Read the model definition and answer for the solid it produces. Units are mm, in the model's axes. Face numbers are marked on the shaded views. A direction names the side the tool comes from. Give positions to 0.01 mm unless a question says otherwise; leave off trailing zeros. Order: outer loops, then holes, each group sorted by start corner. A loop starts at its lowest first (then second) coordinate and runs counter-clockwise, first axis right, second up.
```python
from build123d import *

# Parameters (mm, degrees)
S_BOX1_W       = 20
S_BOX1_H       = 2.5
BOSS_1_DEPTH   = 42
S_BOX2_W       = 30.4
S_BOX2_H       = 24
BOSS_2_DEPTH   = 27.6
S_CUT3_W       = 30.6
S_CUT3_H       = 13
POCKET_3_DEPTH = 23.6
S_CUT4_W       = 23
S_CUT4_H       = 4
POCKET_4_DEPTH = 23.7
S_HOLE5_R      = 1.5
HOLE_5_DEPTH   = 2.7


with BuildPart() as part:
    # S_box1 → Boss_1 (new body)
    with BuildSketch(Plane.XY.offset(-34)):
        with Locations((0, 2.75)):
            Rectangle(S_BOX1_W, S_BOX1_H)
    extrude(amount=BOSS_1_DEPTH)

    # S_box2 → Boss_2 (add)
    with BuildSketch(Plane.XY.offset(-35.4)):
        with Locations((-3.8, 13.5)):
            Rectangle(S_BOX2_W, S_BOX2_H)
    extrude(amount=BOSS_2_DEPTH)

    # S_cut3 → Pocket_3 (cut)
    with BuildSketch(Plane.XY.offset(-33.4)):
        with Locations((-3.8, 17)):
            Rectangle(S_CUT3_W, S_CUT3_H)
    extrude(amount=POCKET_3_DEPTH, mode=Mode.SUBTRACT)

    # S_cut4 → Pocket_4 (cut)
    with BuildSketch(Plane.XY.offset(-35.5)):
        with Locations((-3.5, 6.5)):
            Rectangle(S_CUT4_W, S_CUT4_H)
    extrude(amount=POCKET_4_DEPTH, mode=Mode.SUBTRACT)

    # S_hole5 → Hole_5 (cut)
    with BuildSketch(Plane(origin=(0, 1.4, 0), x_dir=(1, 0, 0), z_dir=(0, 1, 0))):
        with Locations(Location((0, 0, 0), (0, 0, 90))):
            Circle(S_HOLE5_R)
    extrude(amount=HOLE_5_DEPTH, mode=Mode.SUBTRACT)


solid = part.part
```
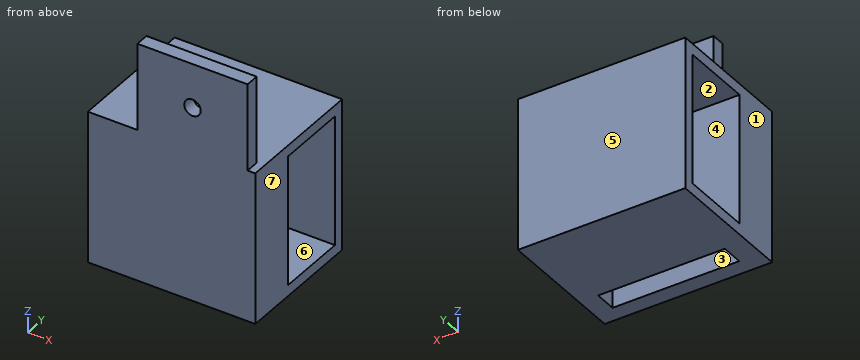
1) The part is cut by section A-A on y = 17. Determine the outline of the cut face in (x, z), and give its area (3 significant figures).
Final values:
outline: (-19, -35.4) - (11.4, -35.4) - (11.4, -33.4) - (-19, -33.4) - close; (-19, -9.8) - (11.4, -9.8) - (11.4, -7.8) - (-19, -7.8) - close
area: 122 mm2
2) The part is cut by section B-B on x = 0. Determine the outline of the cut face in (y, z), and give its area (3 significant figures).
Final values:
outline: (1.5, -35.4) - (4.5, -35.4) - (4.5, -11.8) - (8.5, -11.8) - (8.5, -35.4) - (25.5, -35.4) - (25.5, -7.8) - (4, -7.8) - (4, -1.5) - (1.5, -1.5) - close; (1.5, 1.5) - (4, 1.5) - (4, 8) - (1.5, 8) - close; hole (10.5, -33.4) - (23.5, -33.4) - (23.5, -9.8) - (10.5, -9.8) - close
area: 293 mm2
3) Given pin 1 (4.5 mm diameter, centred on x = -3.5, z = 0.5, fed in from +Y); pin 2 (2 mm diameter, centred on x = -6, y = 6, fed in from -Z); pin 3 (2.5 mm diameter, centred on x = 0, z = 0, fed in from -Y); pin 4 (5 mm diameter, centred on x = -14.5, y = 11.5, fed in from +Z), each flat-ended and moving along its own axis, determine where each tip first touches the part or whether it passes through.
Final values:
pin 1: stops at y = 4
pin 2: stops at z = -11.8
pin 3: passes through
pin 4: stops at z = -7.8
4) The part is cut by section D-D on x = -9. Determine the outline of the cut face in (y, z), and give its area (3 significant figures).
Final values:
outline: (1.5, -35.4) - (4.5, -35.4) - (4.5, -11.8) - (8.5, -11.8) - (8.5, -35.4) - (25.5, -35.4) - (25.5, -7.8) - (4, -7.8) - (4, 8) - (1.5, 8) - close; hole (10.5, -33.4) - (23.5, -33.4) - (23.5, -9.8) - (10.5, -9.8) - close
area: 301 mm2
5) Consider L1, parallel to Y at x = -10.5, z = -25.5; L2, parallel to Y at x = -17, z = -30.5; L3, parallel to X at y = 2.6, z = 0. Determine where each line is inside the solid, lowest interval first.
Final values:
L1: y = 1.5 to 4.5, 8.5 to 10.5, 23.5 to 25.5
L2: y = 1.5 to 10.5, 23.5 to 25.5
L3: x = -10 to -1.5, 1.5 to 10
6) The part is cut by section C-C on z = 0. Determine the outline of the cut face in (x, y).
Final values:
outline: (-10, 1.5) - (-1.5, 1.5) - (-1.5, 4) - (-10, 4) - close; (1.5, 1.5) - (10, 1.5) - (10, 4) - (1.5, 4) - close
7) For a pull along Y with two mould halves and no side action, classify the marked faces 4, 5, 6 and 7 as released by +Y, released by -Y, zero draft, split by the parting line, or undercut.
Final values:
face 4: undercut
face 5: released by +Y
face 6: undercut
face 7: zero draft
8) A tool of negligible diameter and unlimited length cuts with its end or side. For the marked faces 1, 2 and 3, from which of +Z, -Z, +X, -X, +Y, -Y can it reach the whole face along a straight path? Write none if from no direction.
Final values:
face 1: +Z, -Z, -X, +Y, -Y
face 2: +X, -X
face 3: -Z
